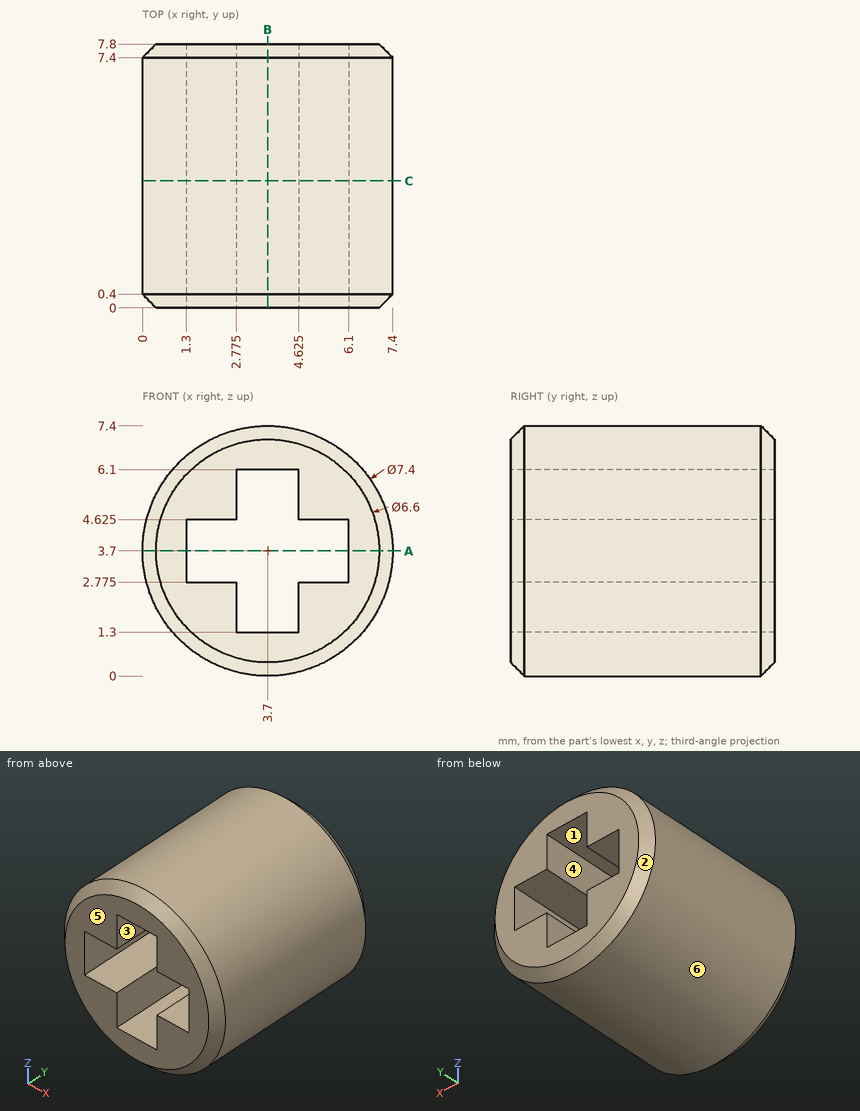
Study the drawing (mm; zero at the part's minimum x, y, z) and answer. A direction names the side the tool comes from. Give positions to 0.01 mm unless a question says otherwise; leave off trailing zeros. Order: outer loops, then holes, each group sorted by start corner. A loop starts at its lowest first (then second) coordinate and runs counter-clockwise, first axis right, second up. Notation, with made-up numbers: (66.5, 43.5) - (116.5, 43.5) arc R18 ccw to (116.5, 57.5) - close; hole circle Ø11 at (54.5, 23). An arc over 180 degrees is marked (long way). Use one line per item in the form item = value. Start each with the question number.
(1) A cutting plane is placed at B-B, the plane x = 3.7. Write down the section's boundary in (y, z).
(2) A cutting plane is placed at A-A, the plane z = 3.7. Write down the section's boundary in (x, y), then the cut area to 3 significant figures.
(3) A cutting plane is placed at C-C, the plane y = 3.75. Write down the section's boundary in (x, z) (3 decimals), then the cut area to 3 significant figures.
(4) For the marked faces 1 and 2, determine the directions among +Z, -Z, +X, -X, +Y, -Y from which every point of the face is accessible in a straight line to the end or side of a thin tool.
(5) Flat-ended cylindrical pins translate along their axes: pin 1 Ø0.9 at (y, z) = (3, 4) entering from +X; pin 2 Ø0.7 at (x, y) = (5.5, 2.5) entering from -Z; pin 3 Ø1.6 at (x, y) = (2.5, 2.5) entering from +Z; pin 4 Ø1 at (x, y) = (6, 5) entering from +Z. Find the tip coordinate at first contact, or state that the pin passes through.
(6) Consider line 1 (Z direction, x = 3.75, y = 4.75); line 2 (X direction, y = 5.5, z = 4.5); line 3 (Z direction, x = 1.75, y = 4.25) (3 decimals). Determine where each line is inside the solid, lowest interval first. Write a range as from..to.
(7) The mould has two halves that part along X. Classify the marked faces 3, 4, 5 and 6: released by +X, released by -X, zero draft, split by the parting line, or undercut.
Ans:
q1.outline = (0, 0.4) - (0.4, 0) - (7.4, 0) - (7.8, 0.4) - (7.8, 1.3) - (0, 1.3) - close; (0, 6.1) - (7.8, 6.1) - (7.8, 7) - (7.4, 7.4) - (0.4, 7.4) - (0, 7) - close
q2.outline = (0, 0.4) - (0.4, 0) - (1.3, 0) - (1.3, 7.8) - (0.4, 7.8) - (0, 7.4) - close; (6.1, 0) - (7, 0) - (7.4, 0.4) - (7.4, 7.4) - (7, 7.8) - (6.1, 7.8) - close
q2.area = 20.0 mm^2
q3.outline = circle Ø7.4 at (3.7, 3.7); hole (1.3, 2.775) - (2.775, 2.775) - (2.775, 1.3) - (4.625, 1.3) - (4.625, 2.775) - (6.1, 2.775) - (6.1, 4.625) - (4.625, 4.625) - (4.625, 6.1) - (2.775, 6.1) - (2.775, 4.625) - (1.3, 4.625) - close
q3.area = 28.7 mm^2
q4.face_1 = +Y, -Y
q4.face_2 = +Y
q5.pin_1 = 7.4
q5.pin_2 = 0.3
q5.pin_3 = 7.38
q5.pin_4 = 6.93
q6.line_1 = 0..1.3, 6.1..7.4
q6.line_2 = 0.09..1.3, 6.1..7.31
q6.line_3 = 0.556..2.775, 4.625..6.844
q7.face_3 = undercut
q7.face_4 = undercut
q7.face_5 = zero draft
q7.face_6 = split by the parting line
